Geometry: final body of the model. Coordinates: model frame, mm. Round coordinates to 2 decimals unless told otherwise and drop trailing zeros. Loops run counter-clockwise (first coordinate to the right, second up) from the corner with the lowest first, then second, coordinate; pieces in that order, holes last. Notation, with made-up numbers: M 67,12 L 102,12 A26 ccw 102,47 Z; hole C -31,31.25 d5. An arc over 180 degrees is marked long. Return JSON: item names as keys, results as strings.
from build123d import *

# Parameters (mm, degrees)
F0_W     = 120
F0_H     = 160
F0_W_2   = 10
F0_H_2   = 10
F1_DEPTH = 25


with BuildPart() as f1:
    # F0 (on Top) → F1 (new body)
    with BuildSketch(Plane.XY):
        Rectangle(F0_W, F0_H)
        with Locations((-50, -70)):
            Rectangle(F0_W_2, F0_H_2, mode=Mode.SUBTRACT)
        with Locations((-50, -50)):
            Rectangle(F0_W_2, F0_H_2, mode=Mode.SUBTRACT)
        with Locations((-30, -70)):
            Rectangle(F0_W_2, F0_H_2, mode=Mode.SUBTRACT)
        with Locations((-10, -70)):
            Rectangle(F0_W_2, F0_H_2, mode=Mode.SUBTRACT)
        with Locations((-30, -50)):
            Rectangle(F0_W_2, F0_H_2, mode=Mode.SUBTRACT)
        with Locations((-10, -50)):
            Rectangle(F0_W_2, F0_H_2, mode=Mode.SUBTRACT)
        with Locations((-50, -30)):
            Rectangle(F0_W_2, F0_H_2, mode=Mode.SUBTRACT)
        with Locations((-50, -10)):
            Rectangle(F0_W_2, F0_H_2, mode=Mode.SUBTRACT)
        with Locations((-30, -30)):
            Rectangle(F0_W_2, F0_H_2, mode=Mode.SUBTRACT)
        with Locations((-10, -30)):
            Rectangle(F0_W_2, F0_H_2, mode=Mode.SUBTRACT)
        with Locations((-30, -10)):
            Rectangle(F0_W_2, F0_H_2, mode=Mode.SUBTRACT)
        with Locations((-10, -10)):
            Rectangle(F0_W_2, F0_H_2, mode=Mode.SUBTRACT)
        with Locations((10, -70)):
            Rectangle(F0_W_2, F0_H_2, mode=Mode.SUBTRACT)
        with Locations((10, -50)):
            Rectangle(F0_W_2, F0_H_2, mode=Mode.SUBTRACT)
        with Locations((30, -70)):
            Rectangle(F0_W_2, F0_H_2, mode=Mode.SUBTRACT)
        with Locations((50, -70)):
            Rectangle(F0_W_2, F0_H_2, mode=Mode.SUBTRACT)
        with Locations((30, -50)):
            Rectangle(F0_W_2, F0_H_2, mode=Mode.SUBTRACT)
        with Locations((50, -50)):
            Rectangle(F0_W_2, F0_H_2, mode=Mode.SUBTRACT)
        with Locations((10, -30)):
            Rectangle(F0_W_2, F0_H_2, mode=Mode.SUBTRACT)
        with Locations((10, -10)):
            Rectangle(F0_W_2, F0_H_2, mode=Mode.SUBTRACT)
        with Locations((30, -30)):
            Rectangle(F0_W_2, F0_H_2, mode=Mode.SUBTRACT)
        with Locations((50, -30)):
            Rectangle(F0_W_2, F0_H_2, mode=Mode.SUBTRACT)
        with Locations((30, -10)):
            Rectangle(F0_W_2, F0_H_2, mode=Mode.SUBTRACT)
        with Locations((50, -10)):
            Rectangle(F0_W_2, F0_H_2, mode=Mode.SUBTRACT)
        with Locations((-50, 10)):
            Rectangle(F0_W_2, F0_H_2, mode=Mode.SUBTRACT)
        with Locations((-50, 30)):
            Rectangle(F0_W_2, F0_H_2, mode=Mode.SUBTRACT)
        with Locations((-30, 10)):
            Rectangle(F0_W_2, F0_H_2, mode=Mode.SUBTRACT)
        with Locations((-10, 10)):
            Rectangle(F0_W_2, F0_H_2, mode=Mode.SUBTRACT)
        with Locations((-30, 30)):
            Rectangle(F0_W_2, F0_H_2, mode=Mode.SUBTRACT)
        with Locations((-10, 30)):
            Rectangle(F0_W_2, F0_H_2, mode=Mode.SUBTRACT)
        with Locations((-50, 50)):
            Rectangle(F0_W_2, F0_H_2, mode=Mode.SUBTRACT)
        with Locations((-50, 70)):
            Rectangle(F0_W_2, F0_H_2, mode=Mode.SUBTRACT)
        with Locations((-30, 50)):
            Rectangle(F0_W_2, F0_H_2, mode=Mode.SUBTRACT)
        with Locations((-10, 50)):
            Rectangle(F0_W_2, F0_H_2, mode=Mode.SUBTRACT)
        with Locations((-30, 70)):
            Rectangle(F0_W_2, F0_H_2, mode=Mode.SUBTRACT)
        with Locations((-10, 70)):
            Rectangle(F0_W_2, F0_H_2, mode=Mode.SUBTRACT)
        with Locations((10, 10)):
            Rectangle(F0_W_2, F0_H_2, mode=Mode.SUBTRACT)
        with Locations((10, 30)):
            Rectangle(F0_W_2, F0_H_2, mode=Mode.SUBTRACT)
        with Locations((30, 10)):
            Rectangle(F0_W_2, F0_H_2, mode=Mode.SUBTRACT)
        with Locations((50, 10)):
            Rectangle(F0_W_2, F0_H_2, mode=Mode.SUBTRACT)
        with Locations((30, 30)):
            Rectangle(F0_W_2, F0_H_2, mode=Mode.SUBTRACT)
        with Locations((50, 30)):
            Rectangle(F0_W_2, F0_H_2, mode=Mode.SUBTRACT)
        with Locations((10, 50)):
            Rectangle(F0_W_2, F0_H_2, mode=Mode.SUBTRACT)
        with Locations((10, 70)):
            Rectangle(F0_W_2, F0_H_2, mode=Mode.SUBTRACT)
        with Locations((30, 50)):
            Rectangle(F0_W_2, F0_H_2, mode=Mode.SUBTRACT)
        with Locations((50, 50)):
            Rectangle(F0_W_2, F0_H_2, mode=Mode.SUBTRACT)
        with Locations((30, 70)):
            Rectangle(F0_W_2, F0_H_2, mode=Mode.SUBTRACT)
        with Locations((50, 70)):
            Rectangle(F0_W_2, F0_H_2, mode=Mode.SUBTRACT)
    extrude(amount=F1_DEPTH)


solid = f1.part
Q1. Pull-direction query (X, two-part tool) for faces 1 (the flat face through (-55, -50, 12)), 2 (the flat face through (10, -65, 12)); classes: pulls with the +X half, pulls with the -X half, needs draft (parallel to the pull), parting line crosses it, or undercut.
Determined:
{"face 1": "undercut", "face 2": "undercut"}
Q2. Section query B-B (x = 12). State how many separate pieces and enclosed holes the cut face has, plus the area to 3 significant figures.
Determined:
{"separate pieces": "9", "enclosed holes": "0", "area": "2,000 mm^2"}
Q3. Section query A-A (y = 48.5). Output: boundary loops of the cut face in (x, z), plus the area to 3 significant figures.
Determined:
{"outline": "M -60,0 L -55,0 L -55,25 L -60,25 Z; M -45,0 L -35,0 L -35,25 L -45,25 Z; M -25,0 L -15,0 L -15,25 L -25,25 Z; M -5,0 L 5,0 L 5,25 L -5,25 Z; M 15,0 L 25,0 L 25,25 L 15,25 Z; M 35,0 L 45,0 L 45,25 L 35,25 Z; M 55,0 L 60,0 L 60,25 L 55,25 Z", "area": "1,500 mm^2"}
Q4. Pin query (flat end, axial travel): pin 1 (6 mm diameter, centred on x = -24, y = 16.5, fed in from -Z). Return the tip coordinate at first contact, or that it passes through.
Determined:
{"pin 1": "stops at z = 0"}
